Source: three-view drawing plus pictorial views. Frame: mm from the lowest corner of the part. Coordinates: 2 decimals unless noted, no trailing zeros. Write each loop counter-clockwise with the first axis right and the second up, starting at its lowest first coordinate (ties: lowest second). Pieces come first, ordered by that corner, then holes. Notation, with made-up numbers: M -10,6 L 16,6 A20 ccw 16,28 Z; hole C 17,-0.5 d9. An arc over 180 degrees is marked long. Write item = value, one per line. Start each with the question number.
Item 1: Ray query, L1, parallel to Z at x = 32.5, y = 1.1; L2, parallel to Z at x = 31.5, y = 0.6; L3, parallel to X at y = 1.4, z = 12.75. Return the intervals inside material, ascending. Write a range as [from, to].
Item 2: Section A-A on x = 32.5. Output: boundary loops of the cut face in (y, z), plus the area to 3 significant figures.
Item 3: Section C-C on x = 2.75. Output: boundary loops of the cut face in (y, z).
Item 4: First-contact query: pin 1 Ø3 at (x, z) = (32.5, 2.25) entering from -Y. Flat tip, straight axial feed; report the tip coordinate or a pass-through.
Item 5: Section B-B on y = 1.25. Output: boundary loops of the cut face in (x, z), plus the area to 3 significant figures.
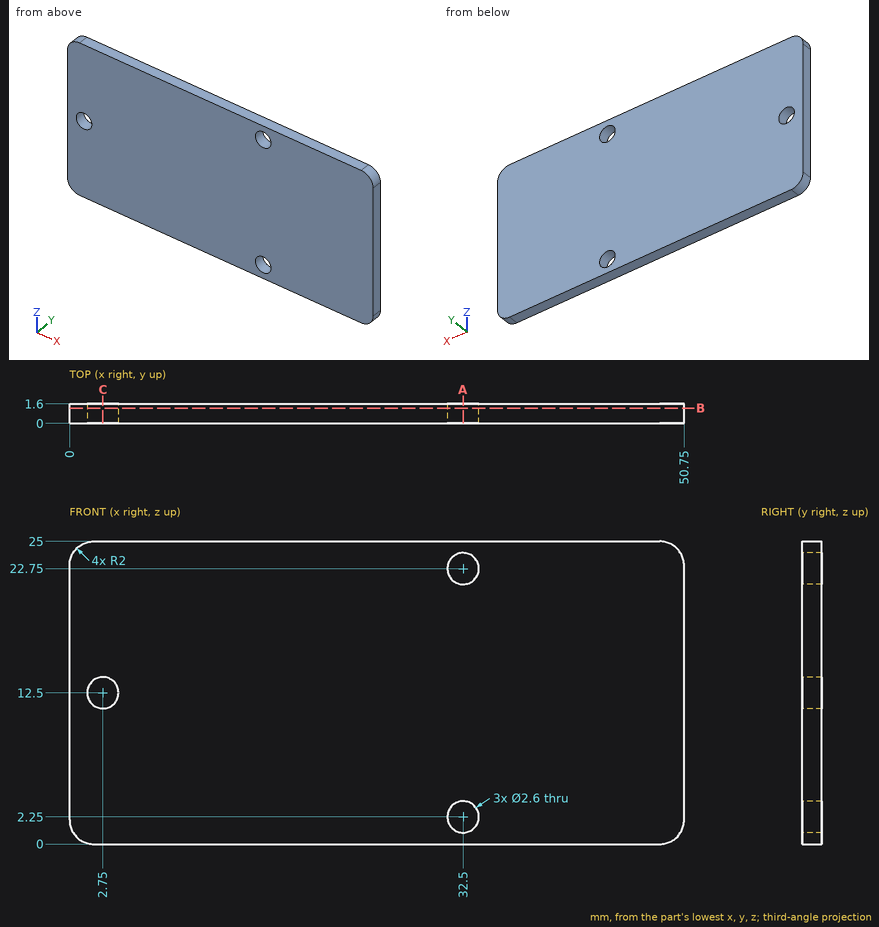
Responses:
q1.L1 = [0, 0.95], [3.55, 21.45], [24.05, 25]
q1.L2 = [0, 1.42], [3.08, 21.92], [23.58, 25]
q1.L3 = [0, 1.47], [4.03, 50.75]
q2.outline = M 0,0 L 1.6,0 L 1.6,0.95 L 0,0.95 Z; M 0,3.55 L 1.6,3.55 L 1.6,21.45 L 0,21.45 Z; M 0,24.05 L 1.6,24.05 L 1.6,25 L 0,25 Z
q2.area = 31.7 mm²
q3.outline = M 0,0 L 1.6,0 L 1.6,11.2 L 0,11.2 Z; M 0,13.8 L 1.6,13.8 L 1.6,25 L 0,25 Z
q4.pin_1 = 0
q5.outline = M 0,2 A2 ccw 2,0 L 48.75,0 A2 ccw 50.75,2 L 50.75,23 A2 ccw 48.75,25 L 2,25 A2 ccw 0,23 Z; hole C 2.75,12.5 d2.6; hole C 32.5,2.25 d2.6; hole C 32.5,22.75 d2.6
q5.area = 1,250 mm²
